Could you check a few things on this model? Use its own coordinates, in mm. Round coordinates to 2 decimals unless told otherwise and drop trailing zeros. Loops run counter-clockwise (first coordinate to the right, second up) from the corner with the lowest first, then second, coordinate; pieces in that order, holes last. Notation, with made-up numbers: (59.25, -32.5) - (74.25, -32.5) arc R24 cw to (74.25, -16.5) - close; hole circle Ø5 at (60, 52). An arc over 180 degrees is marked (long way). Use one line per item in the form item = value.
```python
from build123d import *

# Parameters (mm, degrees)
SKETCH_1_W      = 40
SKETCH_1_H      = 40
SKETCH_1_R      = 2.5
EXTRUDE_3_DEPTH = 5


with BuildPart() as part:
    # 草图1 → 凸台-拉伸3 (new body)
    # profile 1 of 3: a face of its own
    with BuildSketch(Plane(origin=(0, 0, 0), x_dir=(1, 0, 0), z_dir=(0, 1, 0))):
        with BuildLine():
            Line((-100, 10), (-100, -10))
            ThreePointArc((-100, -10), (-97.071067812, -17.071067812), (-90, -20))
            Line((-90, -20), (-20, -20))
            Line((-20, -20), (-20, 20))
            Line((-20, 20), (-90, 20))
            ThreePointArc((-90, 20), (-97.071067812, 17.071067812), (-100, 10))
        make_face()
        with BuildLine():
            ThreePointArc((-70, 5), (-75, 0), (-70, -5))
            Line((-70, -5), (-40, -5))
            ThreePointArc((-40, -5), (-35, 0), (-40, 5))
            Line((-40, 5), (-70, 5))
        make_face(mode=Mode.SUBTRACT)
    # profile 2 of 3: a face of its own
    with BuildSketch(Plane(origin=(0, 0, 0), x_dir=(1, 0, 0), z_dir=(0, 1, 0))):
        Rectangle(SKETCH_1_W, SKETCH_1_H)
        with Locations(Location((0, 0, 0), (0, 0, 270))):
            Circle(SKETCH_1_R, mode=Mode.SUBTRACT)
    # profile 3 of 3: a face of its own
    with BuildSketch(Plane(origin=(0, 0, 0), x_dir=(1, 0, 0), z_dir=(0, 1, 0))):
        with BuildLine():
            ThreePointArc((90, 20), (97.071067812, 17.071067812), (100, 10))
            Line((100, 10), (100, -10))
            ThreePointArc((100, -10), (97.071067812, -17.071067812), (90, -20))
            Line((90, -20), (20, -20))
            Line((20, -20), (20, 20))
            Line((20, 20), (90, 20))
        make_face()
        with BuildLine():
            ThreePointArc((70, -5), (75, 0), (70, 5))
            Line((70, 5), (40, 5))
            ThreePointArc((40, 5), (35, 0), (40, -5))
            Line((40, -5), (70, -5))
        make_face(mode=Mode.SUBTRACT)
    extrude(amount=EXTRUDE_3_DEPTH)


solid = part.part
```
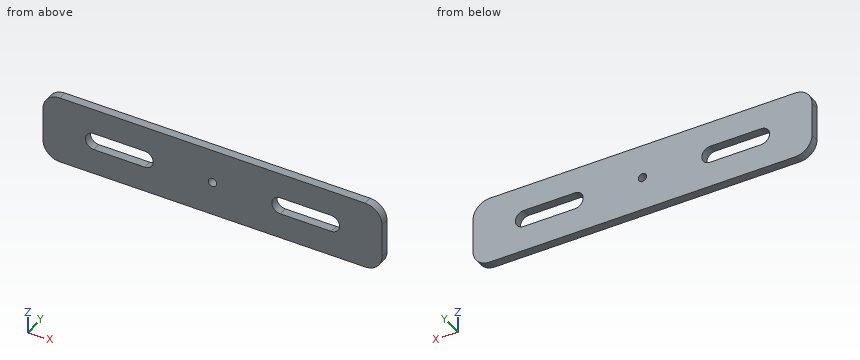
1. If we section it at B-B, the plane z = 0: Write out the boundary of the cut face in (x, y).
Solution:
outline = (-100, 0) - (-75, 0) - (-75, 5) - (-100, 5) - close; (-35, 0) - (-2.5, 0) - (-2.5, 5) - (-35, 5) - close; (2.5, 0) - (35, 0) - (35, 5) - (2.5, 5) - close; (75, 0) - (100, 0) - (100, 5) - (75, 5) - close
2. If we section it at A-A, the plane x = 62: Write out the boundary of the cut face in (y, z), plus the area to 3 significant figures.
Solution:
outline = (0, -20) - (5, -20) - (5, -5) - (0, -5) - close; (0, 5) - (5, 5) - (5, 20) - (0, 20) - close
area = 150 mm^2
3. If we section it at C-C, the plane y = 3.35: Write out the boundary of the cut face in (x, z).
Solution:
outline = (-100, -10) arc R10 ccw to (-90, -20) - (90, -20) arc R10 ccw to (100, -10) - (100, 10) arc R10 ccw to (90, 20) - (-90, 20) arc R10 ccw to (-100, 10) - close; hole (-70, -5) - (-40, -5) arc R5 ccw to (-40, 5) - (-70, 5) arc R5 ccw to start; hole circle Ø5 at (0, 0); hole (40, -5) - (70, -5) arc R5 ccw to (70, 5) - (40, 5) arc R5 ccw to start
4. Please list where these lines run through material, in increasing order: line 1 along X through (y, z) = (2.8, 0); line 2 along Z through (x, y) = (58.5, 1.1); line 3 along X through (y, z) = (1.45, -3).
Solution:
line_1 = -100 to -75, -35 to -2.5, 2.5 to 35, 75 to 100
line_2 = -20 to -5, 5 to 20
line_3 = -100 to -74, -36 to 36, 74 to 100
5. For P1, Ø6, axis at x = 64, z = 14, coming from the -Y side, with a flat end and sliding along its axis, tell me the tip position at first contact or that it passes through.
Solution:
P1 = 0
